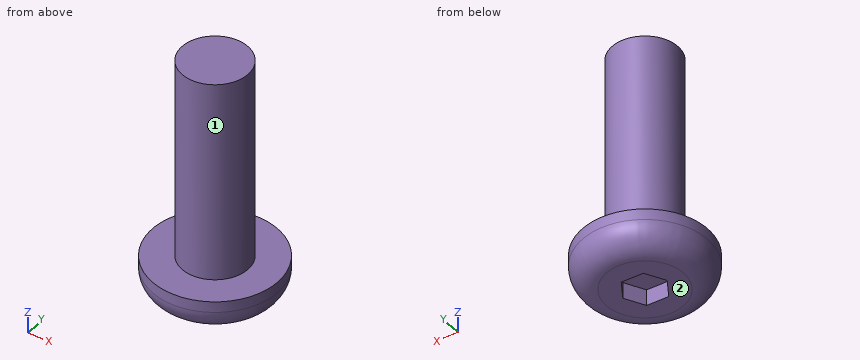
from build123d import *

# Parameters (mm, degrees)
SKETCH1_R      = 3.9624
EXTRUDE1_DEPTH = 2.2098
FILLET1_R      = 1.524
SKETCH2_R      = 2.0828
EXTRUDE2_DEPTH = 12.7
EXTRUDE3_DEPTH = 1.016


with BuildPart() as part:
    # Sketch1 → Extrude1 (new body)
    with BuildSketch(Plane.XY):
        Circle(SKETCH1_R)
    extrude(amount=EXTRUDE1_DEPTH)

    # Fillet1
    fillet1_edges = [part.edges().sort_by_distance(p)[0] for p in [
        (-3.9624, 0, 0),
    ]]
    fillet(fillet1_edges, radius=FILLET1_R)

    # Sketch2 → Extrude2 (add)
    with BuildSketch(Plane.XY.offset(2.2098)):
        Circle(SKETCH2_R)
    extrude(amount=EXTRUDE2_DEPTH)

    # Sketch3 → Extrude3 (cut)
    with BuildSketch(Plane(origin=(0, 0, 0), x_dir=(-1, 0, 0), z_dir=(0, 0, -1))):
        Polygon((0.709024608, 1.177879999), (-0.665561698, 1.202973322), (-1.374586306, 0.025093323), (-0.709024608, -1.177879999), (0.665561698, -1.202973322), (1.374586306, -0.025093323), align=None)
    extrude(amount=-EXTRUDE3_DEPTH, mode=Mode.SUBTRACT)


solid = part.part
Input: part model. Units: mm. Frame: model coordinates. Face numbers are marked on the shaded views. A direction names the side the tool comes from. Give positions to 0.01 mm unless a question says otherwise; leave off trailing zeros. Order: outer loops, then holes, each group sorted by start corner. A loop starts at its lowest first (then second) coordinate and runs counter-clockwise, first axis right, second up. Notation, with made-up numbers: (-35.5, 51.5) -> (1.5, 51.5) arc R16 cw to (1.5, 74.5) -> close; hole circle Ø3 at (54.5, -8.75). An arc over 180 degrees is marked (long way). Use one line per item in the form item = value.
1) Line query: probe 1 along Z at (x, y) = (0.5, 0); probe 2 along Z at (x, y) = (-0.75, 2.25); probe 3 along Y at (x, z) = (-0.75, 0.5). Output: solid intervals per line, ascending.
Response values:
probe_1 = 1.02 to 14.91
probe_2 = 0 to 2.21
probe_3 = -3.49 to -1.06, 1.1 to 3.49
2) Reachability of the marked faces 1 and 2 from +Z, -Z, +X, -X, +Y, -Y: full face, straight path, thin tool, end or side. Return the list, or none.
Response values:
face_1 = +Z
face_2 = -Z, +X, -X, +Y, -Y
3) Section C-C, the plane z = 8.25. Return loops of the section in (x, y).
Response values:
outline = circle Ø4.17 at (0, 0)
4) Section A-A, the plane x = 0. Return loops of the section in (y, z), and give its area (3 significant figures).
Response values:
outline = (-3.96, 1.52) arc R1.52 ccw to (-2.44, 0) -> (-1.19, 0) -> (-1.19, 1.02) -> (1.19, 1.02) -> (1.19, 0) -> (2.44, 0) arc R1.52 ccw to (3.96, 1.52) -> (3.96, 2.21) -> (2.08, 2.21) -> (2.08, 14.91) -> (-2.08, 14.91) -> (-2.08, 2.21) -> (-3.96, 2.21) -> close
area = 67.0 mm^2
5) Section B-B, the plane z = 2. Return loops of the section in (x, y).
Response values:
outline = circle Ø7.92 at (0, 0)
6) First-contact query: pin 1 Ø1 at (x, z) = (-0.5, 5) entering from -Y; pin 2 Ø2 at (y, z) = (-0.5, 6.5) entering from -X; pin 3 Ø3 at (y, z) = (1.5, 11.5) entering from +X. Flat tips, straight axial feed; report the tip coordinate or a pass-through.
Response values:
pin_1 = -2.08
pin_2 = -2.08
pin_3 = 2.08
